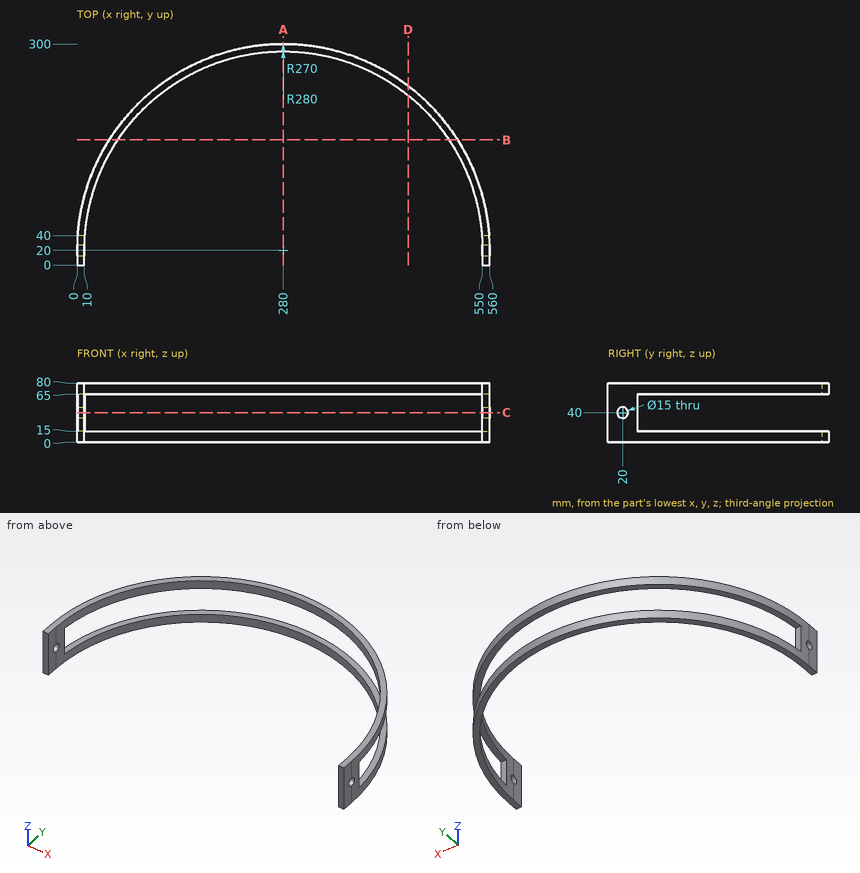
The figure shows three views and two pictorial views of one solid part (mm, origin at its lowest corner). Answer the questions. Coordinates: 2 decimals unless noted, no trailing zeros. Loops run counter-clockwise (first coordinate to the right, second up) from the corner with the lowest first, then second, coordinate; pieces in that order, holes last. Notation, with made-up numbers: (77, 66) - (124, 66) arc R34 ccw to (124, 105) - close; hole circle Ø8 at (45.25, 2.5). An arc over 180 degrees is marked (long way). Answer in a Markdown table with one row per item.
Q1. Find section D-D on x = 449. Write down the section's boundary in (y, z).
Here are the results:
| item | result |
|---|---|
| outline | (230.57, 0) - (243.25, 0) - (243.25, 15) - (230.57, 15) - close; (230.57, 65) - (243.25, 65) - (243.25, 80) - (230.57, 80) - close |
Q2. Find section A-A on x = 280. Write down the section's boundary in (y, z).
Here are the results:
| item | result |
|---|---|
| outline | (290, 0) - (300, 0) - (300, 15) - (290, 15) - close; (290, 65) - (300, 65) - (300, 80) - (290, 80) - close |
Q3. Find section C-C on z = 40. Write down the section's boundary in (x, y), plus the area to 3 significant figures.
Here are the results:
| item | result |
|---|---|
| outline | (0, 0) - (10, 0) - (10, 12.5) - (0, 12.5) - close; (0.1, 27.5) - (10.1, 27.5) arc R270 cw to (10.74, 40) - (0.72, 40) arc R280 ccw to start; (549.26, 40) arc R270 cw to (549.9, 27.5) - (559.9, 27.5) arc R280 ccw to (559.28, 40) - close; (550, 0) - (560, 0) - (560, 12.5) - (550, 12.5) - close |
| area | 500 mm^2 |
Q4. Given P1, Ø12, axis at y = 20, z = 40, coming from the +X side; P2, Ø5, axis at x = 3.5, z = 32.5, coming from the +Y side; P3, Ø10, axis at x = 393.5, z = 14.5, coming from the -Y side, each flat-ended and moving along its own axis, determine where each tip first touches the part or whether it passes through.
Here are the results:
| item | result |
|---|---|
| P1 | passes through |
| P2 | stops at y = 40 |
| P3 | stops at y = 262.61 |
Q5. Straight lines are drawn through the part: line 1 along Z through (x, y) = (3.75, 20); line 2 along Y through (x, z) = (4, 40); line 3 along X through (y, z) = (13, 33.5). For each, find the intervals that lie inside material, in ascending order. Write a range as [from, to].
Here are the results:
| item | result |
|---|---|
| line 1 | z = [0, 32.5], [47.5, 80] |
| line 2 | y = [0, 12.5], [27.5, 40] |
| line 3 | x = [0, 10], [550, 560] |
Q6. Find section B-B on y = 170. Write down the section's boundary in (x, z).
Here are the results:
| item | result |
|---|---|
| outline | (43.57, 0) - (55.5, 0) - (55.5, 15) - (43.57, 15) - close; (43.57, 65) - (55.5, 65) - (55.5, 80) - (43.57, 80) - close; (504.5, 0) - (516.43, 0) - (516.43, 15) - (504.5, 15) - close; (504.5, 65) - (516.43, 65) - (516.43, 80) - (504.5, 80) - close |
